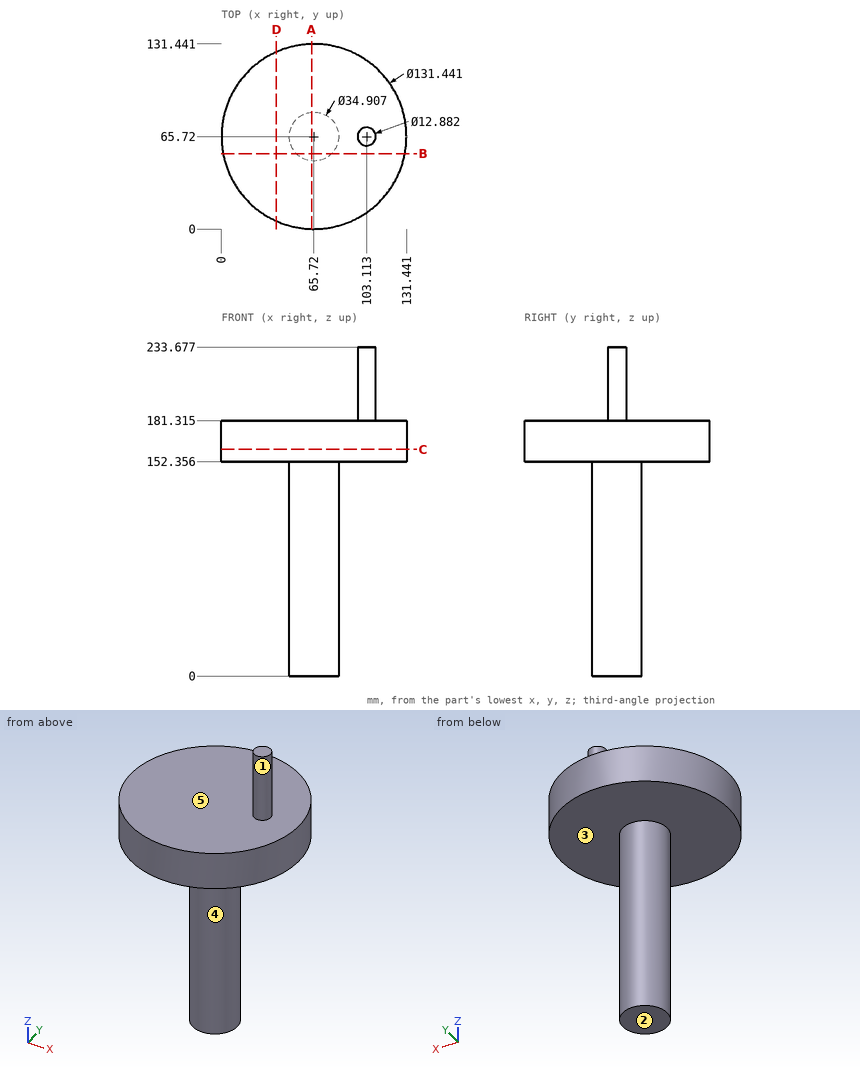
Here's the drawing with two shaded views (mm, measured from the low corner). I have some questions. A direction names the side the tool comes from. Coordinates: 2 decimals unless noted, no trailing zeros. Loops run counter-clockwise (first coordinate to the right, second up) from the corner with the lowest first, then second, coordinate; pieces in that order, holes last. Notation, with made-up numbers: (12.25, 9.5) - (66.25, 9.5) arc R23 ccw to (66.25, 48.5) - close; hole circle Ø6 at (-35.75, 30.25). An arc over 180 degrees is marked (long way). Answer as CSV lines item,"result". Start each with the question number.
1) For pin 1 (4 mm diameter, centred on x = 61, y = 60.5, fed in from +Z) (1 decimal); pin 2 (2 mm diameter, centred on y = 73.5, z = 163.5, fed in from +X); pin 3 (1 mm diameter, centred on x = 19, y = 45, fed in from -Z), each with a flat end and sliding along its axis, tell me the tip position at first contact or that it passes through.
2) Suppose I cut it at C-C (z = 161). Please give me the cut outline in (x, y).
3) I need wall thicknesses on line 1 (Z direction, x = 77, y = 95.5) (1 decimal); line 2 (X direction, y = 56.5, z = 77); line 3 (X direction, y = 62, z = 40.5). Which ranges of each line are inside material? Lowest first, please. Write a range as from..to.
4) Thinking about a two-plate mould opening in X: for the marked faces 4 and 5, which applies, pulls with the +X half, pulls with the -X half, needs draft (parallel to the pull), parting line crosses it, or undercut?
5) Suppose I cut it at D-D (x = 39). Please give me the cut outline in (y, z) (1 decimal).
6) Suppose I cut it at B-B (y = 53.5). Please give me the cut outline in (x, z) (1 decimal).
7) Suppose I cut it at A-A (x = 64). Please give me the cut outline in (y, z) (1 decimal).
8) Which directions (+Z, -Z, +X, -X, +Y, -Y) give clear straight access to the entire face, cutting with the end or side of a thin tool? Please do the marked faces 1, 2 and 3.
Check result:
1,pin 1,"stops at z = 181.3"
1,pin 2,"stops at x = 131.09"
1,pin 3,"stops at z = 152.36"
2,outline,"circle Ø131.44 at (65.72, 65.72)"
3,line 1,"z = 152.4..181.3"
3,line 2,"x = 50.9..80.54"
3,line 3,"x = 48.67..82.77"
4,face 4,"parting line crosses it"
4,face 5,"needs draft"
5,outline,"(5.7, 152.4) - (125.8, 152.4) - (125.8, 181.3) - (5.7, 181.3) - close"
6,outline,"(1.1, 152.4) - (53.3, 152.4) - (53.3, 0) - (78.2, 0) - (78.2, 152.4) - (130.3, 152.4) - (130.3, 181.3) - (1.1, 181.3) - close"
7,outline,"(0, 152.4) - (48.4, 152.4) - (48.4, 0) - (83.1, 0) - (83.1, 152.4) - (131.4, 152.4) - (131.4, 181.3) - (0, 181.3) - close"
8,face 1,"+Z"
8,face 2,"-Z, +X, -X, +Y, -Y"
8,face 3,"-Z"
